Autodesk Inventor part; units mm, degrees
ref_plane "YZ Plane" through (0, 0, 0) normal (1, 0, 0) x (0, 1, 0)
ref_plane "XZ Plane" through (0, 0, 0) normal (0, 1, 0) x (-1, 0, 0)
ref_plane "XY Plane" through (0, 0, 0) normal (0, 0, 1) x (1, 0, 0)
sketch "Sketch1" plane through (0, 0, 0) normal (0, 1, 0) x (-1, 0, 0)
  line L0 (-4.4, -12.5) -> (4.4, -12.5)
  line L1 (6.4, -10.5) -> (6.4, 10.5)
  line L2 (4.4, 12.5) -> (-4.4, 12.5)
  line L3 (-6.4, 10.5) -> (-6.4, -10.5)
  line L4 (-6.4, -12.5) -> (6.4, 12.5) construction
  line L5 (6.4, -12.5) -> (-6.4, 12.5) construction
  line L6 (6.4, 10.5) -> (4.4, 12.5)
  line L7 (-4.4, 12.5) -> (-6.4, 10.5)
  line L8 (6.4, -10.5) -> (4.4, -12.5)
  line L9 (-4.4, -12.5) -> (-6.4, -10.5)
  line L10 (0, 12.5) -> (0, 9.5) construction
  line L11 (-1.15, 12.5) -> (-1.15, 9.5)
  line L12 (1.15, 9.5) -> (1.15, 12.5)
  arc A0 (1.15, 12.5) -> (-1.15, 12.5) centre (0, 12.5) ccw
  arc A1 (-1.15, 9.5) -> (1.15, 9.5) centre (0, 9.5) ccw
  line L13 (0, -12.5) -> (0, -9.5) construction
  line L14 (1.15, -12.5) -> (1.15, -9.5)
  line L15 (-1.15, -9.5) -> (-1.15, -12.5)
  arc A2 (-1.15, -12.5) -> (1.15, -12.5) centre (0, -12.5) ccw
  arc A3 (1.15, -9.5) -> (-1.15, -9.5) centre (0, -9.5) ccw
  point P0 (0, 0)
  point P1 (0, 11)
  point P2 (0, -11)
  dimension "d0" = 25
  dimension "d1" = 12.8
  dimension "d2" = 2
  dimension "d3" = 2
  dimension "d4" = 2
  dimension "d5" = 2
  dimension "d6" = 2
  dimension "d7" = 2
  dimension "d8" = 2
  dimension "d9" = 2
  dimension "d10" = 2.3
  dimension "d11" = 2.3
  dimension "d12" = 3
  dimension "d13" = 3
extrude "Extrusion1" add sketch "Sketch1" along normal blind 1.25 contours L9 L3 L7 L2 L11 A1 L12 L6 L1 L8 L0 L14 A3 L15
sketch "Sketch2" plane through (0, 1.25, 0) normal (0, 1, 0) x (1, 0, 0)
  line L0 (5, 7) -> (-5, 7)
  line L1 (-5, 7) -> (-5, -7)
  line L2 (-5, -7) -> (5, -7)
  line L3 (5, -7) -> (5, 7)
  line L4 (5, 7) -> (-5, -7) construction
  line L5 (-5, 7) -> (5, -7) construction
  point P0 (0, 0)
  dimension "d16" = 10
  dimension "d17" = 14
extrude "Extrusion2" add sketch "Sketch2" along normal blind 10
sketch "Sketch3" plane through (0, 0, 0) normal (0, -1, 0) x (1, 0, 0)
  line L0 (5, 7) -> (-5, 7)
  line L1 (-5, 7) -> (-5, -7)
  line L2 (-5, -7) -> (5, -7)
  line L3 (5, -7) -> (5, 7)
  line L4 (5, 7) -> (-5, -7) construction
  line L5 (-5, 7) -> (5, -7) construction
  point P0 (0, 0)
  dimension "d20" = 10
  dimension "d21" = 14
extrude "Extrusion3" add sketch "Sketch3" along normal blind 14
sketch "Sketch4" plane through (-5, 0, 7) normal (0, 0, 1) x (1, 0, 0)
  line L0 (10, 0) -> (10, -14)
  line L1 (10, -14) -> (0, -10)
  line L2 (0, 0) -> (0, -14)
  line L3 (10, -14) -> (0, -14)
  point P0 (5, 0)
  dimension "d24" = 4
extrude "Extrusion4" cut sketch "Sketch4" against normal through all
equation "\"d3\" = d2"
equation "\"d4\" = d2"
equation "\"d5\" = d4"
equation "\"d6\" = d2"
equation "\"d7\" = d6"
equation "\"d8\" = d2"
equation "\"d9\" = d8"
equation "\"d11\" = d10"
equation "\"d13\" = d12"
properties part number "Molex 1061141150 Fiber-Optic Passthrough"
Design review of the part built by this model. Coordinates are the model's own, in mm. A direction names the side the tool comes from. Round coordinates to 2 decimals unless told otherwise and drop trailing zeros. Write each loop counter-clockwise with the first axis right and the second up, starting at its lowest first coordinate (ties: lowest second). Pieces come first, ordered by that corner, then holes. Notation, with made-up numbers: (86, 82.5) -> (140, 82.5) arc R27 cw to (140, 105.5) -> close; hole circle Ø2 at (67.25, 36.5). An arc over 180 degrees is marked (long way). Write item = value, one per line. Start each with the question number.
1) Mouldability with a two-part tool opening along X and no side actions: class faces 1 (the face through (-1.15, 1, -11)), 2 (the face through (5, 6, 0)), 3 (the face through (1.15, 1, -11)), 4 (the face through (-5, 6, 0)) as +X half, -X half, draft (parallel to the pull), parting line (faces both ways), or undercut.
2) Wall thickness on probe 1 along Z at (x, y) = (2, -1.5); probe 2 along Y at (x, z) = (2.75, -9.75); probe 3 along X at (y, z) = (-1, -5.25): over which ranges is each line inside the solid? List them lowest first. Write a range as from..to.
3) Take a section at C-C, the plane y = 6.5. State the section outline as (x, z) points, plus the area to 3 significant figures.
4) Take a section at A-A, the plane x = -2. State the section outline as (y, z) points.
5) Take a section at D-D, the plane x = -5.5. State the section outline as (y, z) points.
6) Clearance check with flat-ended pins moving along their axes: pin 1 (1 mm diameter, centred on y = 0.5, z = -11.5, fed in from +X); pin 2 (2 mm diameter, centred on x = -1.5, z = 0.5, fed in from -Y); pin 3 (1 mm diameter, centred on y = 3.5, z = -4.5, fed in from -X). State where each tip first meets the part, or that it passes through.
7) Take a section at B-B, the plane z = 6. State the section outline as (x, y) points.
8) Tool access review of faces 5 (the face through (0, 6, 7)), 6 (the face through (5, -7, 0)), 7 (the face through (3, 1, -12.5)), 8 (the face through (-5.4, 0.6, -11.5)), 9 (the face through (0, -5, 7)): name each direction out of +Z, -Z, +X, -X, +Y, -Y from which nothing blocks a thin tool from reaching the whole face with its end or side.
Results list:
q1.face_1 = undercut
q1.face_2 = +X half
q1.face_3 = undercut
q1.face_4 = -X half
q2.probe_1 = -7..7
q2.probe_2 = 0..1.25
q2.probe_3 = -5..5
q3.outline = (-5, -7) -> (5, -7) -> (5, 7) -> (-5, 7) -> close
q3.area = 140 mm²
q4.outline = (-11.2, -7) -> (0, -7) -> (0, -12.5) -> (1.25, -12.5) -> (1.25, -7) -> (11.25, -7) -> (11.25, 7) -> (1.25, 7) -> (1.25, 12.5) -> (0, 12.5) -> (0, 7) -> (-11.2, 7) -> close
q5.outline = (0, -11.4) -> (1.25, -11.4) -> (1.25, 11.4) -> (0, 11.4) -> close
q6.pin_1 = 5.9
q6.pin_2 = -11.8
q6.pin_3 = -5
q7.outline = (-6.4, 0) -> (-5, 0) -> (-5, -10) -> (5, -14) -> (5, 0) -> (6.4, 0) -> (6.4, 1.25) -> (5, 1.25) -> (5, 11.25) -> (-5, 11.25) -> (-5, 1.25) -> (-6.4, 1.25) -> close
q8.face_5 = +Z, +X, -X, +Y
q8.face_6 = +Z, -Z, +X, -Y
q8.face_7 = -Z, +X, -X, +Y, -Y
q8.face_8 = -Z, -X, +Y, -Y
q8.face_9 = +Z, +X, -X, -Y
